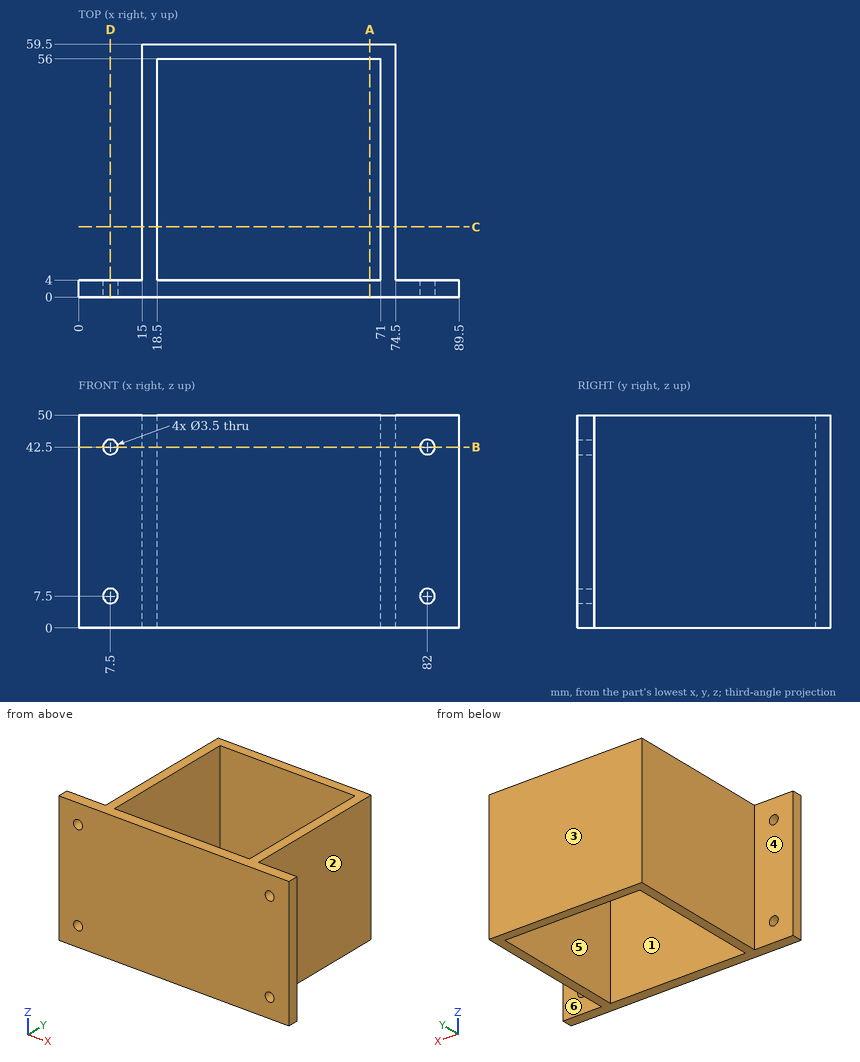
Geometry: see drawing. Coordinates: mm, zero at the bounding-box minimum. A direction names the side the tool comes from. Round coordinates to 2 decimals unless told otherwise and drop trailing zeros. Write each loop counter-clockwise with the first axis right and the second up, starting at its lowest first coordinate (ties: lowest second). Pieces come first, ordered by that corner, then holes. Notation, with made-up numbers: M -9,23 L 3,23 A11 ccw 3,30 Z; hole C 4,17.5 d1. An arc over 180 degrees is marked long. Answer in a Markdown table with one row per item. Add a question column.
(1) Draft query along X for the marked faces 1, 2 and 3. Return one class per face: pulls with the +X half, pulls with the -X half, needs draft (parallel to the pull), parting line crosses it, or undercut.
(2) Cut plane A-A, the plane x = 68.5. Return the cut outline in (y, z), then the cut area to 3 significant figures.
(3) Cut plane D-D, the plane x = 7.5. Return the cut outline in (y, z).
(4) Ray query, L1, parallel to Z at x = 82, y = 1.25; L2, parallel to X at y = 45.5, z = 36.5; L3, parallel to Y at x = 29, z = 44.5. Return the intervals inside material, ascending.
(5) Cut plane C-C, the plane y = 16.5. Return the cut outline in (x, z), then the cut area to 3 significant figures.
(6) Cut plane B-B, the plane z = 42.5. Return the cut outline in (x, y).
(7) Contact query for flat-ended pins moving along their axis: pin 1 (5 mm diameter, centred on y = 12.5, z = 35, fed in from +X); pin 2 (4 mm diameter, centred on x = 7.5, z = 7.5, fed in from +Y); pin 3 (3 mm diameter, centred on x = 82, z = 7.5, fed in from -Y); pin 4 (1.5 mm diameter, centred on y = 9.5, z = 17.5, fed in from -X). Output: stop coordinate, or through.
(8) Reachability of the marked faces 4, 5 and 6 from +Z, -Z, +X, -X, +Y, -Y: full face, straight path, thin tool, end or side. Return the list, or none.
Established:
| question | item | result |
|---|---|---|
| 1 | face 1 | undercut |
| 1 | face 2 | pulls with the +X half |
| 1 | face 3 | needs draft |
| 2 | outline | M 0,0 L 4,0 L 4,50 L 0,50 Z; M 56,0 L 59.5,0 L 59.5,50 L 56,50 Z |
| 2 | area | 375 mm² |
| 3 | outline | M 0,0 L 4,0 L 4,5.75 L 0,5.75 Z; M 0,9.25 L 4,9.25 L 4,40.75 L 0,40.75 Z; M 0,44.25 L 4,44.25 L 4,50 L 0,50 Z |
| 4 | L1 | 0 to 5.75, 9.25 to 40.75, 44.25 to 50 |
| 4 | L2 | 15 to 18.5, 71 to 74.5 |
| 4 | L3 | 0 to 4, 56 to 59.5 |
| 5 | outline | M 15,0 L 18.5,0 L 18.5,50 L 15,50 Z; M 71,0 L 74.5,0 L 74.5,50 L 71,50 Z |
| 5 | area | 350 mm² |
| 6 | outline | M 0,0 L 5.75,0 L 5.75,4 L 0,4 Z; M 9.25,0 L 80.25,0 L 80.25,4 L 74.5,4 L 74.5,59.5 L 15,59.5 L 15,4 L 9.25,4 Z; M 83.75,0 L 89.5,0 L 89.5,4 L 83.75,4 Z; hole M 18.5,4 L 71,4 L 71,56 L 18.5,56 Z |
| 7 | pin 1 | x = 74.5 |
| 7 | pin 2 | y = 4 |
| 7 | pin 3 | through |
| 7 | pin 4 | x = 15 |
| 8 | face 4 | +Z, -Z, -X, +Y |
| 8 | face 5 | +Z, -Z |
| 8 | face 6 | +Z, -Z, +X, +Y |
